Design review of the part built by this model. Coordinates are the model's own, in mm. A direction names the side the tool comes from. Coordinates: 2 decimals unless noted, no trailing zeros. Loops run counter-clockwise (first coordinate to the right, second up) from the corner with the lowest first, then second, coordinate; pieces in that order, holes last. Notation, with made-up numbers: (-28.75, 3.5) - (0.25, 3.5) arc R21 ccw to (0.25, 14.5) - close; hole circle Ø10 at (48, 62). An arc over 180 degrees is marked (long way). Use one line per item in the form item = value. Start each with the question number.
(1) Tool access review of faces 1 (the face through (36.187, -41, 14)), 2 (the face through (36, -42, 19)): name each direction out of +Z, -Z, +X, -X, +Y, -Y from which nothing blocks a thin tool from reaching the whole face with its end or side.
(2) Add section A-A (y = -34). State the section outline as (x, z) points.
(3) For L1, parallel to Y at x = 36.5, z = 12; L2, parallel to X at y = -28, z = 17.25, list the stretches that pass through material, from the lowest coordinate up.
(4) Add section C-C (x = 37.5). State the section outline as (y, z) points, plus the area to 3 significant figures.
(5) Add section B-B (z = 14.75). State the section outline as (x, y) points, plus the area to 3 significant figures.
(6) The part is to be moulded in two halves that separate along X. For faces 3 (the face through (45, -42, 14)), 4 (the face through (38, -20.219, 14)), 5 (the face through (36, -42, 9)), say which applies: pulls with the +X half, pulls with the -X half, needs draft (parallel to the pull), parting line crosses it, or undercut.
```python
from build123d import *

# Parameters (mm, degrees)
SKETCH024_W     = 15
SKETCH024_H     = 65.573825
PAD013_DEPTH    = 10
SKETCH025_W     = 3.980878
SKETCH025_H     = 42.568468
POCKET007_DEPTH = 10.001


with BuildPart() as pocket007:
    # Sketch024 → Pad013 (new body)
    with BuildSketch(Plane(origin=(65, 0, 9), x_dir=(1, 0, 0), z_dir=(0, 0, 1))):
        with Locations((-27.5, 42.000197)):
            Rectangle(SKETCH024_W, SKETCH024_H)
    extrude(amount=PAD013_DEPTH)

    # Sketch025 → Pocket007 (cut, through all)
    with BuildSketch(Plane(origin=(65, 0, 19), x_dir=(1, 0, 0), z_dir=(0, 0, 1))):
        with Locations((-26.822156, 41.502875)):
            Rectangle(SKETCH025_W, SKETCH025_H)
    extrude(amount=-POCKET007_DEPTH, mode=Mode.SUBTRACT)


with BuildPart() as part_mirroring001:
    # Part__Mirroring001: instance of Pocket007
    add(pocket007.part.mirror(Plane(origin=(0, 0, 0), x_dir=(1, 0, 0), z_dir=(0, 1, 0))))


solid = part_mirroring001.part
```
Computed values:
q1.face_1 = +Z, -Z
q1.face_2 = +Z, +X, -X, +Y, -Y
q2.outline = (30, 9) - (36.19, 9) - (36.19, 19) - (30, 19) - close; (40.17, 9) - (45, 9) - (45, 19) - (40.17, 19) - close
q3.L1 = -74.79 to -62.79, -20.22 to -9.21
q3.L2 = 30 to 36.19, 40.17 to 45
q4.outline = (-74.79, 9) - (-62.79, 9) - (-62.79, 19) - (-74.79, 19) - close; (-20.22, 9) - (-9.21, 9) - (-9.21, 19) - (-20.22, 19) - close
q4.area = 230 mm^2
q5.outline = (30, -74.79) - (45, -74.79) - (45, -9.21) - (30, -9.21) - close; hole (36.19, -62.79) - (40.17, -62.79) - (40.17, -20.22) - (36.19, -20.22) - close
q5.area = 814 mm^2
q6.face_3 = pulls with the +X half
q6.face_4 = undercut
q6.face_5 = needs draft
